Check sheet for the modelled part. Datum: model origin and axes. Units: mm. A direction names the side the tool comes from. Round coordinates to 2 decimals unless told otherwise and drop trailing zeros. Loops run counter-clockwise (first coordinate to the right, second up) from the corner with the lowest first, then second, coordinate; pieces in that order, holes last. Notation, with made-up numbers: (88, 51) - (92, 51) arc R14 ccw to (92, 64) - close; hole circle Ø7 at (-10.75, 18.5). An arc over 180 degrees is marked (long way). Answer in a Markdown table with one row per item. Add a question column.
(1) Gauge pin test, flat ends, axial feed: pin 1 (1.5 mm diameter, centred on x = 1, y = 29.5, fed in from -Z); pin 2 (3 mm diameter, centred on y = 28.5, z = 2.5, fed in from -X). Record the tip position at first contact, or that the pin passes through.
(2) Cross-section at B-B on x = 0. Enter the section's corners in (y, z).
(3) Access from +Z, -Z, +X, -X, +Y, -Y to the whole of each face (thin tool, end or side, straight path). Record for faces 1 (the cylindrical face through (-2.373, 44.282, -3.095)), 2 (the flat face through (0, 46, 0)), 3 (the cylindrical face through (-2.373, 1.682, -3.095)).
(4) Cross-section at A-A on z = 0. Enter the section's corners in (x, y).
(5) Cross-section at C-C on y = 24.5. Enter the section's corners in (x, z).
(6) Thickness scan on line 1 along X through (y, z) = (17, -1.5); line 2 along Y through (x, z) = (-0.5, 3.5); line 3 along Z through (x, y) = (-2.25, 35). Record the ranges inside material, lowest first.
from build123d import *

# Parameters (mm, degrees)
SKETCH1_R           = 3.9
BOSS_EXTRUDE1_DEPTH = 46
FILLET5_R           = 0.4
SKETCH2_R           = 4.5
BOSS_EXTRUDE2_DEPTH = 20
CHAMFER1_SIZE       = 0.25


with BuildPart() as part:
    # Sketch1 → Boss-Extrude1 (new body)
    with BuildSketch(Plane(origin=(0, 0, 0), x_dir=(1, 0, 0), z_dir=(0, 1, 0))):
        with Locations(Location((0, 0, 0), (0, 0, 270))):
            Circle(SKETCH1_R)
    extrude(amount=BOSS_EXTRUDE1_DEPTH)

    # Fillet5
    fillet5_edges = [part.edges().sort_by_distance(p)[0] for p in [
        (0, 0, -3.9),
        (0, 46, -3.9),
    ]]
    fillet(fillet5_edges, radius=FILLET5_R)

    # Sketch2 → Boss-Extrude2 (add, symmetric)
    with BuildSketch(Plane(origin=(0, 23, 0), x_dir=(1, 0, 0), z_dir=(0, 1, 0))):
        with Locations(Location((0, 0, 0), (0, 0, 270))):
            Circle(SKETCH2_R)
    extrude(amount=BOSS_EXTRUDE2_DEPTH, both=True)

    # Chamfer1
    chamfer1_edges = [part.edges().sort_by_distance(p)[0] for p in [
        (0, 3, -4.5),
        (0, 43, -4.5),
    ]]
    chamfer(chamfer1_edges, length=CHAMFER1_SIZE)


solid = part.part
Answers:
| question | item | result |
|---|---|---|
| 1 | pin 1 | stops at z = -4.49 |
| 1 | pin 2 | stops at x = -4.39 |
| 2 | outline | (0, -3.5) arc R0.4 ccw to (0.4, -3.9) - (3, -3.9) - (3, -4.25) - (3.25, -4.5) - (42.75, -4.5) - (43, -4.25) - (43, -3.9) - (45.6, -3.9) arc R0.4 ccw to (46, -3.5) - (46, 3.5) arc R0.4 ccw to (45.6, 3.9) - (43, 3.9) - (43, 4.25) - (42.75, 4.5) - (3.25, 4.5) - (3, 4.25) - (3, 3.9) - (0.4, 3.9) arc R0.4 ccw to (0, 3.5) - close |
| 3 | face 1 | +Y |
| 3 | face 2 | +Z, -Z, +X, -X, +Y |
| 3 | face 3 | -Y |
| 4 | outline | (-4.5, 3.25) - (-4.25, 3) - (-3.9, 3) - (-3.9, 0.4) arc R0.4 ccw to (-3.5, 0) - (3.5, 0) arc R0.4 ccw to (3.9, 0.4) - (3.9, 3) - (4.25, 3) - (4.5, 3.25) - (4.5, 42.75) - (4.25, 43) - (3.9, 43) - (3.9, 45.6) arc R0.4 ccw to (3.5, 46) - (-3.5, 46) arc R0.4 ccw to (-3.9, 45.6) - (-3.9, 43) - (-4.25, 43) - (-4.5, 42.75) - close |
| 5 | outline | circle Ø9 at (0, 0) |
| 6 | line 1 | x = -4.24 to 4.24 |
| 6 | line 2 | y = 0 to 46 |
| 6 | line 3 | z = -3.9 to 3.9 |
